from build123d import *

# Parameters (mm, degrees)
F1_DEPTH = 25
F2_DEPTH = 25
F3_DEPTH = 20
F4_R     = 5


with BuildPart() as f1:
    # F0 (on Front) → F1 (new body)
    with BuildSketch(Plane.XZ):
        with BuildLine():
            Line((-40, 40), (0, 0))
            Line((0, 0), (163, 0))
            ThreePointArc((163, 0), (170.071068, 2.928932), (173, 10))
            Line((173, 10), (173, 160))
            Line((173, 160), (133, 200))
            Line((133, 200), (-30, 200))
            ThreePointArc((-30, 200), (-37.071068, 197.071068), (-40, 190))
            Line((-40, 190), (-40, 40))
        make_face()
        with BuildLine():
            Line((112.58571, 9), (37, 9))
            ThreePointArc((37, 9), (29.928932, 11.928932), (27, 19))
            Line((27, 19), (27, 42.421554))
            ThreePointArc((27, 42.421554), (84.312311, 81.209106), (108.629286, 146))
            Line((108.629286, 146), (154, 146))
            ThreePointArc((154, 146), (161.071068, 143.071068), (164, 136))
            Line((164, 136), (164, 79))
            ThreePointArc((164, 79), (161.071068, 71.928932), (154, 69))
            Line((154, 69), (132.48784, 69))
            ThreePointArc((132.48784, 69), (125.416772, 66.071068), (122.48784, 59))
            Line((122.48784, 59), (122.48784, 20.395643))
            ThreePointArc((122.48784, 20.395643), (120.134101, 12.4409), (112.58571, 9))
        make_face(mode=Mode.SUBTRACT)
        with BuildLine():
            ThreePointArc((17.142136, 87.357864), (-11.142136, 87.357864), (-11.142136, 115.642136))
            Line((-11.142136, 115.642136), (57.357864, 184.142136))
            ThreePointArc((57.357864, 184.142136), (85.642136, 184.142136), (85.642136, 155.857864))
            Line((85.642136, 155.857864), (17.142136, 87.357864))
        make_face(mode=Mode.SUBTRACT)
        with BuildLine():
            ThreePointArc((27, 19), (29.928932, 11.928932), (37, 9))
            Line((37, 9), (112.58571, 9))
            ThreePointArc((112.58571, 9), (120.134101, 12.4409), (122.48784, 20.395643))
            Line((122.48784, 20.395643), (122.48784, 59))
            ThreePointArc((122.48784, 59), (125.416772, 66.071068), (132.48784, 69))
            Line((132.48784, 69), (154, 69))
            ThreePointArc((154, 69), (161.071068, 71.928932), (164, 79))
            Line((164, 79), (164, 136))
            ThreePointArc((164, 136), (161.071068, 143.071068), (154, 146))
            Line((154, 146), (108.629286, 146))
            ThreePointArc((108.629286, 146), (84.312311, 81.209106), (27, 42.421554))
            Line((27, 42.421554), (27, 19))
        make_face()
        with BuildLine():
            Line((57.357864, 184.142136), (-11.142136, 115.642136))
            ThreePointArc((-11.142136, 115.642136), (-11.142136, 87.357864), (17.142136, 87.357864))
            Line((17.142136, 87.357864), (85.642136, 155.857864))
            ThreePointArc((85.642136, 155.857864), (85.642136, 184.142136), (57.357864, 184.142136))
        make_face()
        with BuildLine():
            ThreePointArc((64.428932, 177.071068), (78.571068, 177.071068), (78.571068, 162.928932))
            Line((78.571068, 162.928932), (66.323619, 150.681483))
            Line((66.323619, 150.681483), (10.071068, 94.428932))
            ThreePointArc((10.071068, 94.428932), (-4.071068, 94.428932), (-4.071068, 108.571068))
            Line((-4.071068, 108.571068), (52.181483, 164.823619))
            Line((52.181483, 164.823619), (64.428932, 177.071068))
        make_face(mode=Mode.SUBTRACT)
        with BuildLine():
            Line((10.071068, 94.428932), (66.323619, 150.681483))
            ThreePointArc((66.323619, 150.681483), (57.357864, 155.857864), (52.181483, 164.823619))
            Line((52.181483, 164.823619), (-4.071068, 108.571068))
            ThreePointArc((-4.071068, 108.571068), (-4.071068, 94.428932), (10.071068, 94.428932))
        make_face()
        with BuildLine():
            Line((66.323619, 150.681483), (78.571068, 162.928932))
            ThreePointArc((78.571068, 162.928932), (78.571068, 177.071068), (64.428932, 177.071068))
            Line((64.428932, 177.071068), (52.181483, 164.823619))
            ThreePointArc((52.181483, 164.823619), (57.357864, 155.857864), (66.323619, 150.681483))
        make_face()
    extrude(amount=-F1_DEPTH)

    # F0 (on Front) → F2 (join)
    with BuildSketch(Plane.XZ):
        with BuildLine():
            Line((57.357864, 184.142136), (-11.142136, 115.642136))
            ThreePointArc((-11.142136, 115.642136), (-11.142136, 87.357864), (17.142136, 87.357864))
            Line((17.142136, 87.357864), (85.642136, 155.857864))
            ThreePointArc((85.642136, 155.857864), (85.642136, 184.142136), (57.357864, 184.142136))
        make_face()
        with BuildLine():
            ThreePointArc((64.428932, 177.071068), (78.571068, 177.071068), (78.571068, 162.928932))
            Line((78.571068, 162.928932), (66.323619, 150.681483))
            Line((66.323619, 150.681483), (10.071068, 94.428932))
            ThreePointArc((10.071068, 94.428932), (-4.071068, 94.428932), (-4.071068, 108.571068))
            Line((-4.071068, 108.571068), (52.181483, 164.823619))
            Line((52.181483, 164.823619), (64.428932, 177.071068))
        make_face(mode=Mode.SUBTRACT)
    extrude(amount=F2_DEPTH)

    # F0 (on Front) → F3 (cut)
    with BuildSketch(Plane.XZ):
        with BuildLine():
            ThreePointArc((27, 19), (29.928932, 11.928932), (37, 9))
            Line((37, 9), (112.58571, 9))
            ThreePointArc((112.58571, 9), (120.134101, 12.4409), (122.48784, 20.395643))
            Line((122.48784, 20.395643), (122.48784, 59))
            ThreePointArc((122.48784, 59), (125.416772, 66.071068), (132.48784, 69))
            Line((132.48784, 69), (154, 69))
            ThreePointArc((154, 69), (161.071068, 71.928932), (164, 79))
            Line((164, 79), (164, 136))
            ThreePointArc((164, 136), (161.071068, 143.071068), (154, 146))
            Line((154, 146), (108.629286, 146))
            ThreePointArc((108.629286, 146), (84.312311, 81.209106), (27, 42.421554))
            Line((27, 42.421554), (27, 19))
        make_face()
    extrude(amount=-F3_DEPTH, mode=Mode.SUBTRACT)

    # F4
    f4_edges = [f1.edges().sort_by_distance(p)[0] for p in [
        (51.392136, 0, 121.607864),
        (84.312311, 0, 81.209106),
        (84.312311, 20, 81.209106),
        (131.314643, 20, 146),
        (131.314643, 0, 146),
        (27, 0, 30.710777),
        (27, 20, 30.710777),
    ]]
    fillet(f4_edges, radius=F4_R)


solid = f1.part
Work out the finished part from the listing and answer in its coordinate system (mm). A direction names the side the tool comes from. Give positions to 0.01 mm unless a question says otherwise; leave off trailing zeros. Use a Markdown table: item, result. Add a question column.
1. Determine the mould class of faces 4 (the cylindrical face through (-11.45, -14.86, 87.67)), 5 (the cylindrical face through (75, 18, 10)), 6 (the flat face through (50.913, -14.86, 121.128)) for opening direction Z: released by +Z, released by -Z, zero draft, split by the parting line, or undercut.
2. Flat-ended cylindrical pins translate along their axes: pin 1 Ø6 at (x, y) = (60.5, -4) entering from +Z (3 decimals); pin 2 Ø3 at (x, z) = (26.5, 57.5) entering from -Y; pin 3 Ø3 at (x, y) = (147.5, 12.5) entering from +Z. Find the tip coordinate at first contact, or state that the pin passes through.
3. For faces 1 (the cylindrical face through (-3.914, -12.325, 94.275)), 2 (the flat face through (153, 12, 180)), 3 (the flat face through (23.587, -14.86, 150.372)), determine the directions among +Z, -Z, +X, -X, +Y, -Y from which every point of the face is accessible in a straight line to the end or side of a thin tool.
4. Find the intervals of material crossed by probe 1 along X at (y, z) = (15.5, 25); probe 2 along Z at (x, y) = (111, 7); probe 3 along Y at (x, z) = (-27, 133), in increasing order.
Results below:
| question | item | result |
|---|---|---|
| 1 | face 4 | split by the parting line |
| 1 | face 5 | undercut |
| 1 | face 6 | released by -Z |
| 2 | pin 1 | stops at z = 189.355 |
| 2 | pin 2 | stops at y = 0 |
| 2 | pin 3 | stops at z = 187 |
| 3 | face 1 | -Y |
| 3 | face 2 | +Z, +X, +Y, -Y |
| 3 | face 3 | +Z, -X, -Y |
| 4 | probe 1 | x = -25 to 27.03, 122.46 to 173 |
| 4 | probe 2 | z = 0 to 9, 146 to 200 |
| 4 | probe 3 | y = 0 to 25 |
